Geometry check sheet. Reference: the model listing, model coordinates, mm. A direction names the side the tool comes from. Give positions to 0.01 mm unless a question says otherwise; leave off trailing zeros. Loops run counter-clockwise (first coordinate to the right, second up) from the corner with the lowest first, then second, coordinate; pieces in that order, holes last. Notation, with made-up numbers: (-34, 50) -> (-7, 50) arc R21 cw to (-7, 89) -> close; hole circle Ø4 at (20.25, -37.5). An arc over 180 degrees is marked (long way). One line per question, with ' | ' between items.
from build123d import *

# Parameters (mm, degrees)
F0_R     = 1.55
F0_W     = 1.6
F0_H     = 5.1
F1_DEPTH = 1.5
F2_R     = 5
F3_R     = 2
F4_R     = 1


with BuildPart() as f1:
    # F0 (on Top) → F1 (new body)
    with BuildSketch(Plane.XY):
        Polygon((-16.45, -30.5), (16.45, -30.5), (16.45, 10.5), (16.45, 30.5), (11.95, 30.5), (11.95, 19.5), (-11.95, 19.5), (-11.95, 30.5), (-16.45, 30.5), (-16.45, 10.5), align=None)
        with Locations((-14.2, -26.5)):
            Circle(F0_R, mode=Mode.SUBTRACT)
        with Locations((-10, -19.5)):
            Circle(F0_R, mode=Mode.SUBTRACT)
        with Locations((14.2, -26.5)):
            Circle(F0_R, mode=Mode.SUBTRACT)
        with Locations((10, -19.5)):
            Circle(F0_R, mode=Mode.SUBTRACT)
        with Locations((-14.2, 7.5)):
            Circle(F0_R, mode=Mode.SUBTRACT)
        with Locations((-10, 0.5)):
            Circle(F0_R, mode=Mode.SUBTRACT)
        with Locations((-14.2, 14.05)):
            Rectangle(F0_W, F0_H, mode=Mode.SUBTRACT)
        with Locations((-14.2, 24.95)):
            Rectangle(F0_W, F0_H, mode=Mode.SUBTRACT)
        with Locations((10, 0.5)):
            Circle(F0_R, mode=Mode.SUBTRACT)
        with Locations((14.2, 7.5)):
            Circle(F0_R, mode=Mode.SUBTRACT)
        with Locations((14.2, 14.05)):
            Rectangle(F0_W, F0_H, mode=Mode.SUBTRACT)
        with Locations((14.2, 24.95)):
            Rectangle(F0_W, F0_H, mode=Mode.SUBTRACT)
        Polygon((16.45, 10.5), (16.45, -30.5), (18.45, -28.5), (18.45, 8.5), align=None)
        Polygon((-18.45, -28.5), (-16.45, -30.5), (-16.45, 10.5), (-18.45, 8.5), align=None)
    extrude(amount=F1_DEPTH)

    # F2
    f2_edges = [f1.edges().sort_by_distance(p)[0] for p in [
        (-11.95, 19.5, 0.75),
        (11.95, 19.5, 0.75),
    ]]
    fillet(f2_edges, radius=F2_R)

    # F3
    f3_edges = [f1.edges().sort_by_distance(p)[0] for p in [
        (16.45, -30.5, 0.75),
        (18.45, -28.5, 0.75),
        (-18.45, -28.5, 0.75),
        (-16.45, -30.5, 0.75),
        (-18.45, 8.5, 0.75),
        (-16.45, 10.5, 0.75),
        (16.45, 10.5, 0.75),
        (18.45, 8.5, 0.75),
    ]]
    fillet(f3_edges, radius=F3_R)

    # F4
    f4_edges = [f1.edges().sort_by_distance(p)[0] for p in [
        (16.45, 30.5, 0.75),
        (11.95, 30.5, 0.75),
        (-11.95, 30.5, 0.75),
        (-16.45, 30.5, 0.75),
    ]]
    fillet(f4_edges, radius=F4_R)


solid = f1.part
Item 1: Sectioned sample at C-C (x = 10). Record the cut outline in (y, z).
Result:
outline: (-30.5, 0) -> (-21.05, 0) -> (-21.05, 1.5) -> (-30.5, 1.5) -> close; (-17.95, 0) -> (-1.05, 0) -> (-1.05, 1.5) -> (-17.95, 1.5) -> close; (2.05, 0) -> (20.54, 0) -> (20.54, 1.5) -> (2.05, 1.5) -> close
Item 2: Scan lines: probe 1 along X at (y, z) = (26.5, 0.95); probe 2 along Y at (x, z) = (-14, 0.25); probe 3 along X at (y, z) = (16, 0.8). Record each from-to range of solid material in increasing order.
Result:
probe 1: -16.45 to -15, -13.4 to -11.95, 11.95 to 13.4, 15 to 16.45 | probe 2: -30.5 to -28.04, -24.96 to 5.96, 9.04 to 11.5, 16.6 to 22.4, 27.5 to 30.5 | probe 3: -16.45 to -15, -13.4 to 13.4, 15 to 16.45
Item 3: Depth check by flat-ended pin: pin 1 Ø0.8 at (y, z) = (26, 1) entering from -X; pin 2 Ø0.8 at (y, z) = (26, 0.5) entering from +X. Enter the tip coordinate at first touch or a pass-through.
Result:
pin 1: x = -16.45 | pin 2: x = 16.45
Item 4: Sectioned sample at B-B (x = 14.2). Record the cut outline in (y, z), plus the area to 3 significant figures.
Result:
outline: (-30.5, 0) -> (-28.05, 0) -> (-28.05, 1.5) -> (-30.5, 1.5) -> close; (-24.95, 0) -> (5.95, 0) -> (5.95, 1.5) -> (-24.95, 1.5) -> close; (9.05, 0) -> (11.5, 0) -> (11.5, 1.5) -> (9.05, 1.5) -> close; (16.6, 0) -> (22.4, 0) -> (22.4, 1.5) -> (16.6, 1.5) -> close; (27.5, 0) -> (30.5, 0) -> (30.5, 1.5) -> (27.5, 1.5) -> close | area: 66.9 mm2
Item 5: Release check for a two-part mould opening along Y. For faces 4 (the face through (-15, 25, 1)), 5 (the face through (18.3, -28.43, 0.76)), 6 (the face through (0, 19.5, 1)) record: pulls with the +Y half, pulls with the -Y half, needs draft (parallel to the pull), parting line crosses it, or undercut.
Result:
face 4: undercut | face 5: pulls with the -Y half | face 6: pulls with the +Y half
Item 6: Set-up check for faces 1 (the face through (-18.294, -28.447, 0.76)), 2 (the face through (11.95, 27, 1)), 3 (the face through (-13.4, 25, 1)): record each of +Z, -Z, +X, -X, +Y, -Y from which the full face is reachable in a straight line by a thin tool's end or side.
Result:
face 1: +Z, -Z, -X, -Y | face 2: +Z, -Z, +Y | face 3: +Z, -Z
Item 7: Sectioned sample at A-A (y = 0.5). Record the cut outline in (x, z).
Result:
outline: (-18.45, 0) -> (-11.55, 0) -> (-11.55, 1.5) -> (-18.45, 1.5) -> close; (-8.45, 0) -> (8.45, 0) -> (8.45, 1.5) -> (-8.45, 1.5) -> close; (11.55, 0) -> (18.45, 0) -> (18.45, 1.5) -> (11.55, 1.5) -> close
Item 8: Sectioned sample at D-D (z = 0.45). Give the number of separate pieces and of enclosed holes in the cut face, plus the area to 3 significant figures.
Result:
separate pieces: 1 | enclosed holes: 12 | area: 1,820 mm2
